Could you check a few things on this model? Use its own coordinates, in mm. Give positions to 0.01 mm unless a question says otherwise; leave off trailing zeros. Write each loop counter-clockwise with the first axis right and the second up, starting at its lowest first coordinate (ties: lowest second). Pieces come first, ordered by that corner, then holes. Notation, with made-up numbers: M -30,-5 L -14,-5 A19 cw -14,14 Z; hole C 36,60.5 d10. An arc over 180 degrees is marked long. One line per item, written item: value.
```python
from build123d import *

# Parameters (mm, degrees)
BOSS_EXTRUDE1_DEPTH = 1066.8


with BuildPart() as part:
    # Sketch2 → Boss-Extrude1 (new body, symmetric)
    with BuildSketch(Plane.XY):
        Polygon((-6.35, 0), (6.35, 0), (6.35, 12.7), (3.175, 12.7), (3.175, 3.175), (-6.35, 3.175), align=None)
    extrude(amount=BOSS_EXTRUDE1_DEPTH, both=True)


solid = part.part
```
1) I'm going to push flat-ended pins straight in: pin 1 (5 mm diameter, centred on y = 8.5, z = 511, fed in from -X) (3 decimals); pin 2 (3 mm diameter, centred on x = -2, z = 95, fed in from +Y) (3 decimals). Where does each tip first touch, or does it pass through?
Outcome:
pin 1: stops at x = 3.175
pin 2: stops at y = 3.175
2) If we section it at A-A, the plane z = 470.5: Write out the boundary of the cut face in (x, y) (3 decimals).
Outcome:
outline: M -6.35,0 L 6.35,0 L 6.35,12.7 L 3.175,12.7 L 3.175,3.175 L -6.35,3.175 Z
3) Please list where these lines run through material, in increasing order: L1, parallel to X at y = 4, z = -941.5 (3 decimals); L2, parallel to Y at x = 1.5, z = 588 (3 decimals). Write a range as from..to.
Outcome:
L1: x = 3.175..6.35
L2: y = 0..3.175
4) If we section it at C-C, the plane y = 10: Write out the boundary of the cut face in (x, z) (3 decimals), then the cut area to 3 significant figures.
Outcome:
outline: M 3.175,-1066.8 L 6.35,-1066.8 L 6.35,1066.8 L 3.175,1066.8 Z
area: 6,770 mm^2
5) If we section it at B-B, the plane x = 1: Write out the boundary of the cut face in (y, z) (3 decimals), then the cut area to 3 significant figures.
Outcome:
outline: M 0,-1066.8 L 3.175,-1066.8 L 3.175,1066.8 L 0,1066.8 Z
area: 6,770 mm^2
